Read the model definition and answer for the solid it produces. Units are mm, in the model's axes. A direction names the side the tool comes from. Give positions to 0.01 mm unless a question says otherwise; leave off trailing zeros. Order: outer loops, then holes, each group sorted by start corner. A loop starts at its lowest first (then second) coordinate and runs counter-clockwise, first axis right, second up. Notation, with made-up numbers: M -29,52 L -10,52 A20 ccw -10,83 Z; hole C 5,35.25 d5. An arc over 180 degrees is marked long. One line per item, written item: value.
Autodesk Inventor part; units mm, degrees
ref_plane "YZ Plane" through (0, 0, 0) normal (1, 0, 0) x (0, 1, 0)
ref_plane "XZ Plane" through (0, 0, 0) normal (0, 1, 0) x (-1, 0, 0)
ref_plane "XY Plane" through (0, 0, 0) normal (0, 0, 1) x (1, 0, 0)
sketch "Sketch1" plane through (0, 0, 0) normal (0, 0, 1) x (1, 0, 0)
  line L0 (0, 0) -> (18.0086, 0)
  line L1 (18.0086, 0) -> (18.0086, 18.0086)
  line L2 (18.0086, 18.0086) -> (0, 18.0086)
  line L3 (0, 18.0086) -> (0, 0)
  dimension "d0" = 18.0086
  dimension "d1" = 18.0086
extrude "Extrusion1" add sketch "Sketch1" along normal blind 1.27
sketch "Sketch2" plane through (0, 18.0086, 0) normal (0, 1, 0) x (1, 0, 0)
  line L0 (0, 0) -> (18.0086, 0)
  line L1 (18.0086, 0) -> (18.0086, 6.35)
  line L2 (18.0086, 6.35) -> (0, 6.35)
  line L3 (0, 6.35) -> (0, 0)
  dimension "d4" = 6.35
extrude "Extrusion2" add sketch "Sketch2" along normal blind 1.27
sketch "Sketch3" plane through (0, 18.0086, 1.27) normal (0, 1, 0) x (1, 0, 0)
  line L0 (18.0086, 0) -> (0, 0)
  line L1 (0, 0) -> (18.0086, 0)
  line L2 (18.0086, 0) -> (18.0086, 1.27)
  line L3 (18.0086, 1.27) -> (0, 1.27)
  line L4 (0, 1.27) -> (0, 0)
  point P0 (0, 1.27)
extrude "Extrusion3" add sketch "Sketch3" along normal blind 1.27
properties part number "CapLiftHolder"
1) Find section B-B, the plane x = 11.75. Write down the section's boundary in (y, z), plus the area to 3 significant figures.
Reported:
outline: M 0,0 L 18.01,0 L 18.01,-6.35 L 19.28,-6.35 L 19.28,1.27 L 0,1.27 Z
area: 32.5 mm^2
2) Each of these flat-tipped pins is pushed along its axis until it touches: pin 1 Ø8 at (x, y) = (7, 8.5) entering from -Z; pin 2 Ø2 at (y, z) = (14.5, -2.5) entering from +X; pin 3 Ø1.9 at (x, z) = (10, -2) entering from -Y. Where does it stop, or does it pass through?
Reported:
pin 1: stops at z = 0
pin 2: passes through
pin 3: stops at y = 18.01
3) Which of the six approach directions +Z, -Z, +X, -X, +Y, -Y give full straight-line access (tool end or side, diameter ignored) to faces 1 (the face through (9, 18.009, -3)), 2 (the face through (0, 12.5, 0.3))?
Reported:
face 1: -Z, +X, -X, -Y
face 2: +Z, -Z, -X, +Y, -Y
4) Consider probe 1 along Y at (x, z) = (2, -3.75); probe 2 along Z at (x, y) = (6.5, 2). Determine where each line is inside the solid, lowest interval first.
Reported:
probe 1: y = 18.01 to 19.28
probe 2: z = 0 to 1.27
5) Find section A-A, the plane y = 12.25. Write down the section's boundary in (x, z).
Reported:
outline: M 0,0 L 18.01,0 L 18.01,1.27 L 0,1.27 Z
6) Find section C-C, the plane z = -0.5. Write down the section's boundary in (x, y).
Reported:
outline: M 0,18.01 L 18.01,18.01 L 18.01,19.28 L 0,19.28 Z
